Design review of the part built by this model. Coordinates are the model's own, in mm. A direction names the side the tool comes from. Coordinates: 2 decimals unless noted, no trailing zeros. Loops run counter-clockwise (first coordinate to the right, second up) from the corner with the lowest first, then second, coordinate; pieces in that order, holes last. Notation, with made-up numbers: (47.5, 6) - (68.5, 6) arc R24 cw to (68.5, 20) - close; hole circle Ø3 at (67.25, -23.75). An arc over 180 degrees is marked (long way). Answer in a Markdown table with one row per item. Add a question column.
(1) For faces 1 (the face through (19, -7, 2)), 2 (the face through (51.557, -95.002, 2.768)), 3 (the face through (30, 0.25, 2)), list the 3-axis set-ups (+Z, -Z, +X, -X, +Y, -Y) from which the entire face can be reached by the end or side of a thin tool; tool diameter is ignored.
(2) We need section B-B, the plane z = 0.6. Give the number of separate pieces and of enclosed holes in the cut face, plus the area to 3 significant figures.
(3) To check wall thickness, follow L1, parallel to X at y = -10, z = 0.45; L2, parallel to X at y = -66, z = 3.2; L3, parallel to Y at x = 7.5, z = 3.8. State the ranges of each line that lie inside material, in increasing order. Write a range as [from, to].
(4) The part is to be moulded in two halves that separate along Y. For faces 4 (the face through (12, -97.6, 2)), 5 (the face through (13.95, -84.395, 2.768)), 6 (the face through (-0.25, -12, 2)), 7 (the face through (57, 0.25, 2)), say which applies: released by +Y, released by -Y, zero draft, split by the parting line, or undercut.
(5) We need section A-A, the plane y = -48. Write out the cut boundary in (x, z), plus the area to 3 significant figures.
(6) Clearance check with flat-ended pins moving along their axes: pin 1 (2 mm diameter, centred on x = 47, z = 2.5, fed in from +Y); pin 2 (3 mm diameter, centred on x = 53, y = -22, fed in from +Z); pin 3 (1 mm diameter, centred on x = 39, z = 1.5, fed in from -Y). State where each tip first meets the part, or that it passes through.
from build123d import *

# Parameters (mm, degrees)
SKETCH1_W           = 5
SKETCH1_H           = 15
SKETCH1_R           = 0.55
SKETCH1_R_2         = 3.5
BOSS_EXTRUDE1_DEPTH = 4
SKETCH2_R           = 1.8
CUT_EXTRUDE1_DEPTH  = 2.5
SKETCH4_R           = 1.8
CUT_EXTRUDE2_DEPTH  = 131.110049573
FILLET1_R           = 5
FILLET2_R           = 2.5
FILLET3_R           = 1.5
FILLET4_R           = 1.5


with BuildPart() as part:
    # Sketch1 → Boss-Extrude1 (new body)
    with BuildSketch(Plane.XY):
        Polygon((5.00009906, -115.25), (5.00009906, -111.60004858), (5.00009906, -97.60004858), (19.00009906, -97.60004858), (19.00009906, -111.60004858), (19.00009906, -115.25), (39.43509906, -115.25), (39.43509906, -111.60004858), (39.43509906, -97.60004858), (53.43509906, -97.60004858), (53.43509906, -111.60004858), (53.43509906, -115.25), (60.25, -115.25), (60.25, 0.25), (54.00009906, 0.25), (54.00009906, -3.50006858), (54.00009906, -17.50006858), (40.00009906, -17.50006858), (40.00009906, -3.50006858), (40.00009906, 0.25), (19.00009906, 0.25), (19.00009906, -3.50006858), (19.00009906, -17.50006858), (5.00009906, -17.50006858), (5.00009906, -3.50006858), (5.00009906, 0.25), (-0.25, 0.25), (-0.25, -24.5), (4.5, -24.5), (9.5, -24.5), (9.5, -41.5), (9.5, -56.5), (4.5, -56.5), (-0.25, -56.5), (-0.25, -115.25), align=None)
        with Locations((7, -87)):
            Rectangle(SKETCH1_W, SKETCH1_H, mode=Mode.SUBTRACT)
        with Locations((15.686582595, -91.313399625)):
            Circle(SKETCH1_R, mode=Mode.SUBTRACT)
        with Locations((19.99993396, -87.00004826)):
            Circle(SKETCH1_R_2, mode=Mode.SUBTRACT)
        with Locations((24.313285325, -82.686696895)):
            Circle(SKETCH1_R, mode=Mode.SUBTRACT)
        with Locations((42.686582595, -91.313399625)):
            Circle(SKETCH1_R, mode=Mode.SUBTRACT)
        with Locations((46.99993396, -87.00004826)):
            Circle(SKETCH1_R_2, mode=Mode.SUBTRACT)
        with Locations((35.186582595, -61.686696895)):
            Circle(SKETCH1_R, mode=Mode.SUBTRACT)
        with Locations((39.49993396, -66.00004826)):
            Circle(SKETCH1_R_2, mode=Mode.SUBTRACT)
        with Locations((43.813285325, -70.313399625)):
            Circle(SKETCH1_R, mode=Mode.SUBTRACT)
        with Locations((51.313285325, -82.686696895)):
            Circle(SKETCH1_R, mode=Mode.SUBTRACT)
        with Locations((51.313285325, -31.313399625)):
            Circle(SKETCH1_R, mode=Mode.SUBTRACT)
        with Locations((42.686582595, -22.686696895)):
            Circle(SKETCH1_R, mode=Mode.SUBTRACT)
        with Locations((46.99993396, -27.00004826)):
            Circle(SKETCH1_R_2, mode=Mode.SUBTRACT)
    extrude(amount=BOSS_EXTRUDE1_DEPTH)

    # Sketch2 → Cut-Extrude1 (cut)
    # profile 1 of 8: a face of its own
    with BuildSketch(Plane.XY.offset(4)):
        Polygon((26.140038593, -95.42634332), (28.42622902, -93.140152893), (27.589425245, -90.017158692), (24.466431045, -89.180354918), (22.180240618, -91.466545345), (23.017044392, -94.589539545), align=None)
        with Locations((25.303234819, -92.303349119)):
            Circle(SKETCH2_R, mode=Mode.SUBTRACT)
    # profile 2 of 8: a face of its own
    with BuildSketch(Plane.XY.offset(4)):
        Polygon((13.859829327, -78.5737532), (11.5736389, -80.859943627), (12.410442675, -83.982937828), (15.533436875, -84.819741602), (17.819627302, -82.533551175), (16.982823528, -79.410556975), align=None)
        with Locations((14.696633101, -81.696747401)):
            Circle(SKETCH2_R, mode=Mode.SUBTRACT)
    # profile 3 of 8: a face of its own
    with BuildSketch(Plane.XY.offset(4)):
        Polygon((53.140038593, -95.42634332), (55.42622902, -93.140152893), (54.589425245, -90.017158692), (51.466431045, -89.180354918), (49.180240618, -91.466545345), (50.017044392, -94.589539545), align=None)
        with Locations((52.303234819, -92.303349119)):
            Circle(SKETCH2_R, mode=Mode.SUBTRACT)
    # profile 4 of 8: a face of its own
    with BuildSketch(Plane.XY.offset(4)):
        Polygon((38.5736389, -80.859943627), (39.410442675, -83.982937828), (42.533436875, -84.819741602), (44.819627302, -82.533551175), (43.982823528, -79.410556975), (40.859829327, -78.5737532), align=None)
        with Locations((41.696633101, -81.696747401)):
            Circle(SKETCH2_R, mode=Mode.SUBTRACT)
    # profile 5 of 8: a face of its own
    with BuildSketch(Plane.XY.offset(4)):
        Polygon((31.0736389, -72.140152893), (33.359829327, -74.42634332), (36.482823528, -73.589539545), (37.319627302, -70.466545345), (35.033436875, -68.180354918), (31.910442675, -69.017158692), align=None)
        with Locations((34.196633101, -71.303349119)):
            Circle(SKETCH2_R, mode=Mode.SUBTRACT)
    # profile 6 of 8: a face of its own
    with BuildSketch(Plane.XY.offset(4)):
        Polygon((47.92622902, -59.859943627), (45.640038593, -57.5737532), (42.517044392, -58.410556975), (41.680240618, -61.533551175), (43.966431045, -63.819741602), (47.089425245, -62.982937828), align=None)
        with Locations((44.803234819, -60.696747401)):
            Circle(SKETCH2_R, mode=Mode.SUBTRACT)
    # profile 7 of 8: a face of its own
    with BuildSketch(Plane.XY.offset(4)):
        Polygon((44.819627302, -31.466545345), (42.533436875, -29.180354918), (39.410442675, -30.017158692), (38.5736389, -33.140152893), (40.859829327, -35.42634332), (43.982823528, -34.589539545), align=None)
        with Locations((41.696633101, -32.303349119)):
            Circle(SKETCH2_R, mode=Mode.SUBTRACT)
    # profile 8 of 8: a face of its own
    with BuildSketch(Plane.XY.offset(4)):
        Polygon((54.589425245, -23.982937828), (55.42622902, -20.859943627), (53.140038593, -18.5737532), (50.017044392, -19.410556975), (49.180240618, -22.533551175), (51.466431045, -24.819741602), align=None)
        with Locations((52.303234819, -21.696747401)):
            Circle(SKETCH2_R, mode=Mode.SUBTRACT)
    extrude(amount=-CUT_EXTRUDE1_DEPTH, mode=Mode.SUBTRACT)

    # Sketch4 → Cut-Extrude2 (cut, through all)
    with BuildSketch(Plane.XY.offset(4)):
        with Locations((52.303234819, -21.696747401)):
            Circle(SKETCH4_R)
        with Locations((41.696633101, -32.303349119)):
            Circle(SKETCH4_R)
        with Locations((44.803234819, -60.696747401)):
            Circle(SKETCH4_R)
        with Locations((34.196633101, -71.303349119)):
            Circle(SKETCH4_R)
        with Locations((41.696633101, -81.696747401)):
            Circle(SKETCH4_R)
        with Locations((52.303234819, -92.303349119)):
            Circle(SKETCH4_R)
        with Locations((25.303234819, -92.303349119)):
            Circle(SKETCH4_R)
        with Locations((14.696633101, -81.696747401)):
            Circle(SKETCH4_R)
    extrude(amount=-CUT_EXTRUDE2_DEPTH, mode=Mode.SUBTRACT)

    # Fillet1
    fillet1_edges = [part.edges().sort_by_distance(p)[0] for p in [
        (53.43509906, -97.60004858, 2),
        (39.43509906, -97.60004858, 2),
        (19.00009906, -97.60004858, 2),
        (5.00009906, -97.60004858, 2),
        (5.00009906, -17.50006858, 2),
        (19.00009906, -17.50006858, 2),
        (40.00009906, -17.50006858, 2),
        (54.00009906, -17.50006858, 2),
    ]]
    fillet(fillet1_edges, radius=FILLET1_R)

    # Fillet2
    fillet2_edges = [part.edges().sort_by_distance(p)[0] for p in [
        (9.5, -56.5, 2),
        (9.5, -24.5, 2),
    ]]
    fillet(fillet2_edges, radius=FILLET2_R)

    # Fillet3
    fillet3_edges = [part.edges().sort_by_distance(p)[0] for p in [
        (4.5, -94.5, 2),
        (9.5, -94.5, 2),
        (9.5, -79.5, 2),
        (4.5, -79.5, 2),
    ]]
    fillet(fillet3_edges, radius=FILLET3_R)

    # Fillet4
    fillet4_edges = [part.edges().sort_by_distance(p)[0] for p in [
        (60.25, 0.25, 2),
        (60.25, -115.25, 2),
        (53.43509906, -115.25, 2),
        (39.43509906, -115.25, 2),
        (19.00009906, -115.25, 2),
        (5.00009906, -115.25, 2),
        (-0.25, -115.25, 2),
        (-0.25, -56.5, 2),
        (-0.25, -24.5, 2),
        (-0.25, 0.25, 2),
        (5.00009906, 0.25, 2),
        (19.00009906, 0.25, 2),
        (40.00009906, 0.25, 2),
        (54.00009906, 0.25, 2),
    ]]
    fillet(fillet4_edges, radius=FILLET4_R)


solid = part.part
Responses:
| question | item | result |
|---|---|---|
| 1 | face 1 | +Z, -Z, +Y |
| 1 | face 2 | +Z |
| 1 | face 3 | +Z, -Z, +X, -X, +Y |
| 2 | separate pieces | 1 |
| 2 | enclosed holes | 21 |
| 2 | area | 5,410 mm2 |
| 3 | L1 | x = [-0.25, 5], [19, 40], [54, 60.25] |
| 3 | L2 | x = [-0.25, 36], [43, 60.25] |
| 3 | L3 | y = [-98.27, -94.5], [-79.5, -56.45], [-24.55, -16.83] |
| 4 | face 4 | released by -Y |
| 4 | face 5 | undercut |
| 4 | face 6 | zero draft |
| 4 | face 7 | released by +Y |
| 5 | outline | (9.5, 0) - (60.25, 0) - (60.25, 4) - (9.5, 4) - close |
| 5 | area | 203 mm2 |
| 6 | pin 1 | stops at y = -17.5 |
| 6 | pin 2 | stops at z = 1.5 |
| 6 | pin 3 | stops at y = -115.14 |
